Part print with two shaded views. Sizes in mm from the minimum x, y, z corner. A direction names the side the tool comes from. Coordinates: 2 decimals unless noted, no trailing zeros. Loops run counter-clockwise (first coordinate to the right, second up) from the corner with the lowest first, then second, coordinate; pieces in that order, holes last. Notation, with made-up numbers: (-29, -39.75) -> (-2, -39.75) arc R30 ccw to (-2, -0.75) -> close; hole circle Ø6 at (71.5, 30.25). An arc over 180 degrees is marked (long way). Return JSON: item names as keys, results as strings. Group by question number.
(1) Mould opens along Y. For the marked faces 4, 5, 6 and 7 say: pulls with the +Y half, pulls with the -Y half, needs draft (parallel to the pull), parting line crosses it, or undercut.
(2) Saw through at C-C on x = 16.5. Write the cut outline in (y, z).
(3) Saw through at B-B on y = 12. Write the cut outline in (x, z).
(4) Probe L1, parallel to Z at x = 38, y = 10.5; L2, parallel to X at y = 0.7, z = 7.5; L3, parallel to Z at x = 10.5, y = 7.5. List the from-to ranges inside material, lowest first.
(5) Saw through at A-A on x = 12. Write the cut outline in (y, z).
(6) Flat gauge pins, fed straight in: pin 1 Ø4 at (x, y) = (12, 9) entering from -Z; pin 2 Ø1.5 at (x, z) = (5, 4) entering from +Y; pin 3 Ø1.6 at (x, z) = (4.07, 7.5) entering from +Y; pin 4 Ø1.5 at (y, z) = (11, 5.5) entering from -X. Where does each tip first touch, or does it go through?
(7) Tool access for the marked faces 1, 2 and 3: list every direction of +Z, -Z, +X, -X, +Y, -Y with a clear straight run to the whole face (end or side of a thin tool).
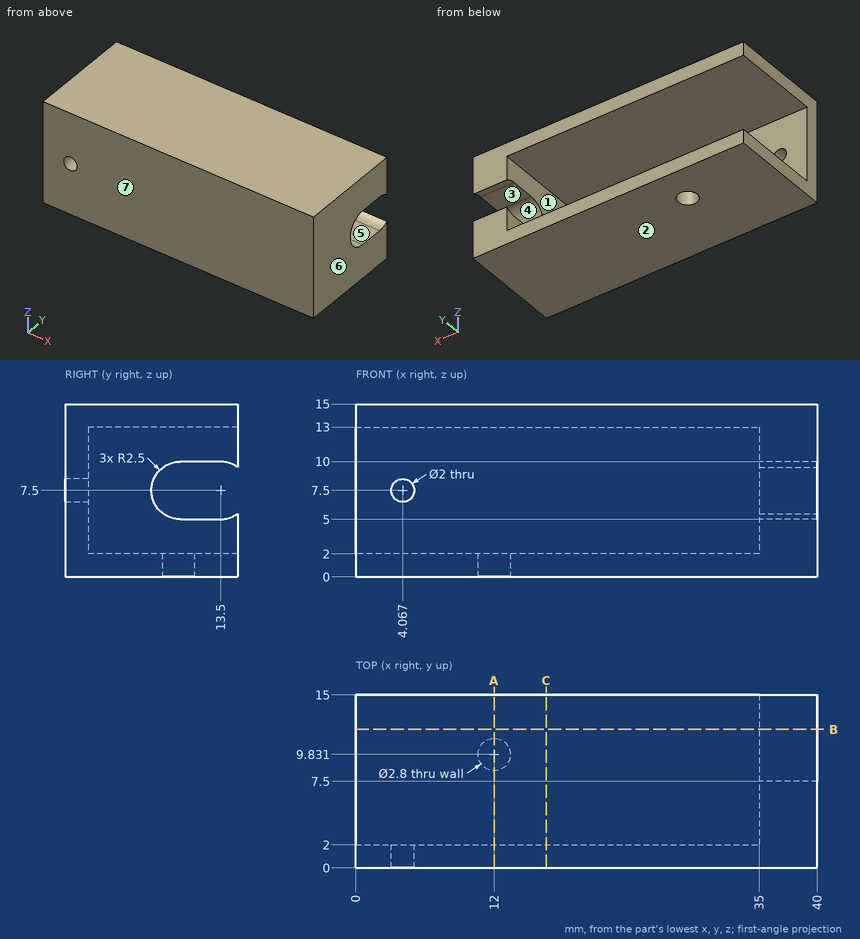
Geometry results:
{
 "1": {"face 4": "undercut", "face 5": "undercut", "face 6": "needs draft", "face 7": "pulls with the -Y half"},
 "2": {"outline": "(0, 0) -> (15, 0) -> (15, 2) -> (2, 2) -> (2, 13) -> (15, 13) -> (15, 15) -> (0, 15) -> close"},
 "3": {"outline": "(0, 0) -> (40, 0) -> (40, 5) -> (35, 5) -> (35, 2) -> (0, 2) -> close; (0, 13) -> (35, 13) -> (35, 10) -> (40, 10) -> (40, 15) -> (0, 15) -> close"},
 "4": {"L1": "0 to 5, 10 to 15", "L2": "0 to 3.07, 5.07 to 40", "L3": "0 to 2, 13 to 15"},
 "5": {"outline": "(0, 0) -> (8.43, 0) -> (8.43, 2) -> (2, 2) -> (2, 13) -> (15, 13) -> (15, 15) -> (0, 15) -> close; (11.23, 0) -> (15, 0) -> (15, 2) -> (11.23, 2) -> close"},
 "6": {"pin 1": "z = 0", "pin 2": "y = 2", "pin 3": "through", "pin 4": "x = 35"},
 "7": {"face 1": "-X, +Y", "face 2": "-Z, +X, -X, +Y, -Y", "face 3": "+X, -X"}
}
